```python
from build123d import *

# Parameters (mm, degrees)
F0_W     = 50.8
F0_H     = 50.8
F0_R     = 8.001
F1_DEPTH = 26.67
F2_W     = 30.48
F2_H     = 50.8
F2_W_2   = 50.8
F2_R     = 8.001
F3_DEPTH = 49.53
F4_R     = 3.2385
F5_DEPTH = 81.281


with BuildPart() as f1:
    # F0 (on Top) → F1 (new body)
    with BuildSketch(Plane.XY):
        Rectangle(F0_W, F0_H)
        Circle(F0_R, mode=Mode.SUBTRACT)
    extrude(amount=F1_DEPTH)

    # F2 (on face) → F3 (join)
    with BuildSketch(Plane.XY.offset(26.67)):
        with Locations((-40.64, 0)):
            Rectangle(F2_W, F2_H)
        Rectangle(F2_W_2, F2_H)
        Circle(F2_R, mode=Mode.SUBTRACT)
        with Locations((40.64, 0)):
            Rectangle(F2_W, F2_H)
    extrude(amount=F3_DEPTH)

    # F4 (on face) → F5 (cut, through all)
    with BuildSketch(Plane(origin=(-25.4, 0, 0), x_dir=(0, -1, 0), z_dir=(-1, 0, 0))):
        with Locations((0, 9.525)):
            Circle(F4_R)
    extrude(amount=-F5_DEPTH, mode=Mode.SUBTRACT)


solid = f1.part
```
The listing builds one solid part. Answer for the finished solid, in the listing's coordinates (mm). A direction names the side the tool comes from. Round coordinates to 2 decimals unless told otherwise and drop trailing zeros. Loops run counter-clockwise (first coordinate to the right, second up) from the corner with the lowest first, then second, coordinate; pieces in that order, holes last. Notation, with made-up numbers: (6.5, 8.5) -> (51.5, 8.5) arc R13 ccw to (51.5, 29.5) -> close; hole circle Ø4 at (-24, 12.5). An arc over 180 degrees is marked (long way). Use one line per item in the form item = value.
1. Flat-ended cylindrical pins translate along their axes: pin 1 Ø24.5 at (x, y) = (41, -10.5) entering from -Z; pin 2 Ø21.5 at (y, z) = (-5.5, 8.5) entering from +X; pin 3 Ø7.5 at (y, z) = (0, 9.525) entering from -X. Find the tip coordinate at first contact, or state that the pin passes through.
Answer key:
pin_1 = 26.67
pin_2 = 25.4
pin_3 = -25.4
2. The part is cut by section A-A on x = 0. Determine the outline of the cut face in (y, z).
Answer key:
outline = (-25.4, 0) -> (-8, 0) -> (-8, 76.2) -> (-25.4, 76.2) -> close; (8, 0) -> (25.4, 0) -> (25.4, 76.2) -> (8, 76.2) -> close
3. A tool of negligible diameter and unlimited length cuts with its end or side. For faces 5 (the flat face through (-25.4, 0, 13)), 6 (the flat face through (-1, -25.4, 46)), 7 (the flat face through (40, 0, 26.67)), from which of +Z, -Z, +X, -X, +Y, -Y can it reach the whole face along a straight path? Write none if from no direction.
Answer key:
face_5 = -Z, -X, +Y, -Y
face_6 = +Z, -Z, +X, -X, -Y
face_7 = -Z, +X, +Y, -Y
4. Find the intervals of material crossed by probe 1 along Z at (x, y) = (-19.25, 0); probe 2 along Y at (x, z) = (-9, 9.5); probe 3 along X at (y, z) = (0, 58), in increasing order. Write a range as [from, to].
Answer key:
probe_1 = [0, 6.29], [12.76, 76.2]
probe_2 = [-25.4, -3.24], [3.24, 25.4]
probe_3 = [-55.88, -8], [8, 55.88]
5. The part is cut by section D-D on y = 13. Determine the outline of the cut face in (x, z).
Answer key:
outline = (-55.88, 26.67) -> (-25.4, 26.67) -> (-25.4, 0) -> (25.4, 0) -> (25.4, 26.67) -> (55.88, 26.67) -> (55.88, 76.2) -> (-55.88, 76.2) -> close
6. The part is cut by section B-B on y = 0. Determine the outline of the cut face in (x, z), and give its area (3 significant figures).
Answer key:
outline = (-55.88, 26.67) -> (-25.4, 26.67) -> (-25.4, 12.76) -> (-8, 12.76) -> (-8, 76.2) -> (-55.88, 76.2) -> close; (-25.4, 0) -> (-8, 0) -> (-8, 6.29) -> (-25.4, 6.29) -> close; (8, 0) -> (25.4, 0) -> (25.4, 6.29) -> (8, 6.29) -> close; (8, 12.76) -> (25.4, 12.76) -> (25.4, 26.67) -> (55.88, 26.67) -> (55.88, 76.2) -> (8, 76.2) -> close
area = 5,450 mm²
7. For a pull along Z with two mould halves and no side action, classify faces 1 (the cylindrical face through (-16.485, 0.702, 6.364)), 2 (the flat face through (-41, 0, 26.67)), 3 (the flat face through (1, 25.4, 46)), 4 (the flat face through (-1, -11, 76.2)) as released by +Z, released by -Z, zero draft, split by the parting line, or undercut.
Answer key:
face_1 = undercut
face_2 = released by -Z
face_3 = zero draft
face_4 = released by +Z
8. The part is cut by section C-C on z = 56.5. Determine the outline of the cut face in (x, y), and give its area (3 significant figures).
Answer key:
outline = (-55.88, -25.4) -> (55.88, -25.4) -> (55.88, 25.4) -> (-55.88, 25.4) -> close; hole circle Ø16 at (0, 0)
area = 5,480 mm²
